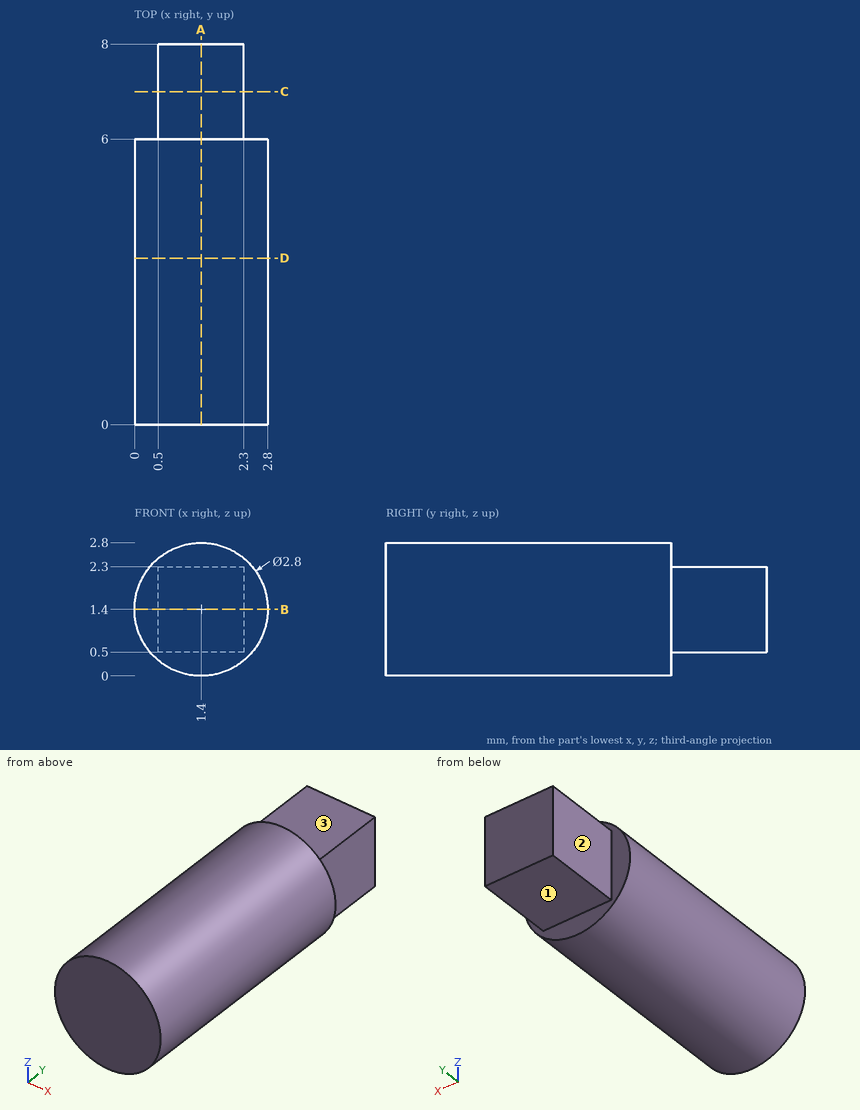
Geometry check sheet. Reference: drawing and pictorial views, mm from the part's lowest x, y, z. A direction names the side the tool comes from. Coordinates: 2 decimals unless noted, no trailing zeros. Order: outer loops, then holes, each group sorted by start corner. A loop starts at its lowest first (then second) coordinate and runs counter-clockwise, first axis right, second up.
Item 1: Section check B-B, the plane z = 1.4. Enter the section's corners in (x, y), then the cut area to 3 significant figures.
Filled in:
outline: (0, 0) - (2.8, 0) - (2.8, 6) - (2.3, 6) - (2.3, 8) - (0.5, 8) - (0.5, 6) - (0, 6) - close
area: 20.4 mm2
Item 2: Section check D-D, the plane y = 3.5. Enter the section's corners in (x, z), then the cut area to 3 significant figures.
Filled in:
outline: circle Ø2.8 at (1.4, 1.4)
area: 6.16 mm2
Item 3: Section check C-C, the plane y = 7. Enter the section's corners in (x, z).
Filled in:
outline: (0.5, 0.5) - (2.3, 0.5) - (2.3, 2.3) - (0.5, 2.3) - close
Item 4: Material ranges on L1, parallel to X at y = 7.25, z = 2.15; L2, parallel to Y at x = 0.4, z = 1.2, recorded low to high.
Filled in:
L1: x = 0.5 to 2.3
L2: y = 0 to 6
Item 5: Section check A-A, the plane x = 1.4. Enter the section's corners in (y, z), then the cut area to 3 significant figures.
Filled in:
outline: (0, 0) - (6, 0) - (6, 0.5) - (8, 0.5) - (8, 2.3) - (6, 2.3) - (6, 2.8) - (0, 2.8) - close
area: 20.4 mm2
Item 6: Depth check by flat-ended pin: pin 1 (0.5 mm diameter, centred on x = 1.5, y = 7, fed in from -Z); pin 2 (0.9 mm diameter, centred on y = 7, z = 1.5, fed in from +X). Enter the tip coordinate at first touch or a pass-through.
Filled in:
pin 1: stops at z = 0.5
pin 2: stops at x = 2.3
Item 7: Access from +Z, -Z, +X, -X, +Y, -Y to the whole of each face (thin tool, end or side, straight path). Record for the marked faces 1, 2 and 3.
Filled in:
face 1: -Z, +X, -X, +Y
face 2: +Z, -Z, -X, +Y
face 3: +Z, +X, -X, +Y
